CAD build for the part. Positions are in the model's coordinates, mm. A direction names the side the tool comes from. Coordinates: 2 decimals unless noted, no trailing zeros. Order: outer loops, then holes, each group sorted by start corner. A loop starts at its lowest first (then second) coordinate and runs counter-clockwise, first axis right, second up. Notation, with made-up numbers: M -12.75,71.25 L 0.25,71.25 A18 cw 0.25,80.25 Z; hole C -28,-13.75 d6. An arc over 180 degrees is marked long. One line per item, written item: value.
from build123d import *

# Parameters (mm, degrees)
SKETCH1_R           = 4.2
SKETCH1_R_2         = 2.2
BOSS_EXTRUDE1_DEPTH = 10
SKETCH2_R           = 4.2
BOSS_EXTRUDE2_DEPTH = 2
SKETCH3_R           = 2.1
BOSS_EXTRUDE3_DEPTH = 15


with BuildPart() as part:
    # Sketch1 → Boss-Extrude1 (new body)
    with BuildSketch(Plane.XY):
        Circle(SKETCH1_R)
        Circle(SKETCH1_R_2, mode=Mode.SUBTRACT)
    extrude(amount=BOSS_EXTRUDE1_DEPTH)

    # Sketch2 → Boss-Extrude2 (add)
    with BuildSketch(Plane.XY.offset(10)):
        Circle(SKETCH2_R)
    extrude(amount=BOSS_EXTRUDE2_DEPTH)

    # Sketch3 → Boss-Extrude3 (add)
    with BuildSketch(Plane.XY.offset(12)):
        Circle(SKETCH3_R)
    extrude(amount=BOSS_EXTRUDE3_DEPTH)


solid = part.part
Q1. Pin check, flat tips, straight feed: pin 1 Ø4 at (y, z) = (-3, 20.5) entering from +X; pin 2 Ø5 at (y, z) = (0.5, 22.5) entering from +X. Stop position of each tip, or through.
Recorded:
pin 1: stops at x = 1.85
pin 2: stops at x = 2.1
Q2. Slice it at A-A (x = 0). List the corners of the cut face in (y, z), plus the area to 3 significant figures.
Recorded:
outline: M -4.2,0 L -2.2,0 L -2.2,10 L 2.2,10 L 2.2,0 L 4.2,0 L 4.2,12 L 2.1,12 L 2.1,27 L -2.1,27 L -2.1,12 L -4.2,12 Z
area: 120 mm^2
Q3. Slice it at D-D (y = -3.5). List the corners of the cut face in (x, z).
Recorded:
outline: M -2.32,0 L 2.32,0 L 2.32,12 L -2.32,12 Z
Q4. Mould opens along Y. For faces 1 (the face through (0, 0, 27)), 2 (the face through (0, 0, 10)), 3 (the face through (2.003, 0.631, 19.395)) say: released by +Y, released by -Y, zero draft, split by the parting line, or undercut.
Recorded:
face 1: zero draft
face 2: undercut
face 3: split by the parting line
Q5. Which spindle directions (+Z, -Z, +X, -X, +Y, -Y) get a long thin tool onto all of the face, cutting with end or side? Do faces 4 (the face through (4.006, 1.262, 5.916)), 5 (the face through (2.1, 0.66, 4.93)), 6 (the face through (2, -2, 12)). Say none if no direction does.
Recorded:
face 4: +Z, -Z
face 5: -Z
face 6: +Z
Q6. Drill centre lines: line 1 along Y through (x, z) = (0, 6.25); line 2 along Z through (x, y) = (0.25, -0.5); line 3 along Z through (x, y) = (2.25, -1.75). Where is each one in solid material? Low to high.
Recorded:
line 1: y = -4.2 to -2.2, 2.2 to 4.2
line 2: z = 10 to 27
line 3: z = 0 to 12
Q7. Slice it at C-C (z = 12.75). List the corners of the cut face in (x, y).
Recorded:
outline: C 0,0 d4.2
